Geometry: see drawing. Coordinates: mm, zero at the bounding-box minimum. Coordinates: 2 decimals unless noted, no trailing zeros. Write each loop counter-clockwise with the first axis right and the second up, starting at its lowest first coordinate (ties: lowest second). Pieces come first, ordered by that corner, then holes. Notation, with made-up numbers: (-0.5, -33) - (40.5, -33) arc R20 cw to (40.5, -13) - close; hole circle Ø6 at (-35, -21.75). An arc over 180 degrees is marked (long way). Use a Markdown table: item, result. Add a question column.
Q1. Section query B-B (z = 1). Return the cut outline in (x, y) (1 decimal).
Q2. Section query A-A (z = 4). Return the cut outline in (x, y) (1 decimal), then the cut area to 3 significant figures.
Q3. Section query C-C (y = 2.25). Return the cut outline in (x, z).
Q4. Section query D-D (x = 1.5). Return the cut outline in (y, z), then the cut area to 3 significant figures.
Q5. Material intervals for probe 1 along X at (y, z) = (14.25, 7.5); probe 2 along X at (y, z) = (14, 1.5); probe 3 along Y at (x, z) = (17, 1) (1 decimal), sorted ascending. Write a range as from..to.
Q6. Mould query, pull axis X, two halves, no side actions, for the marked faces 1, 2 and 3. Classes: released by +X, released by -X, zero draft, split by the parting line, or undercut.
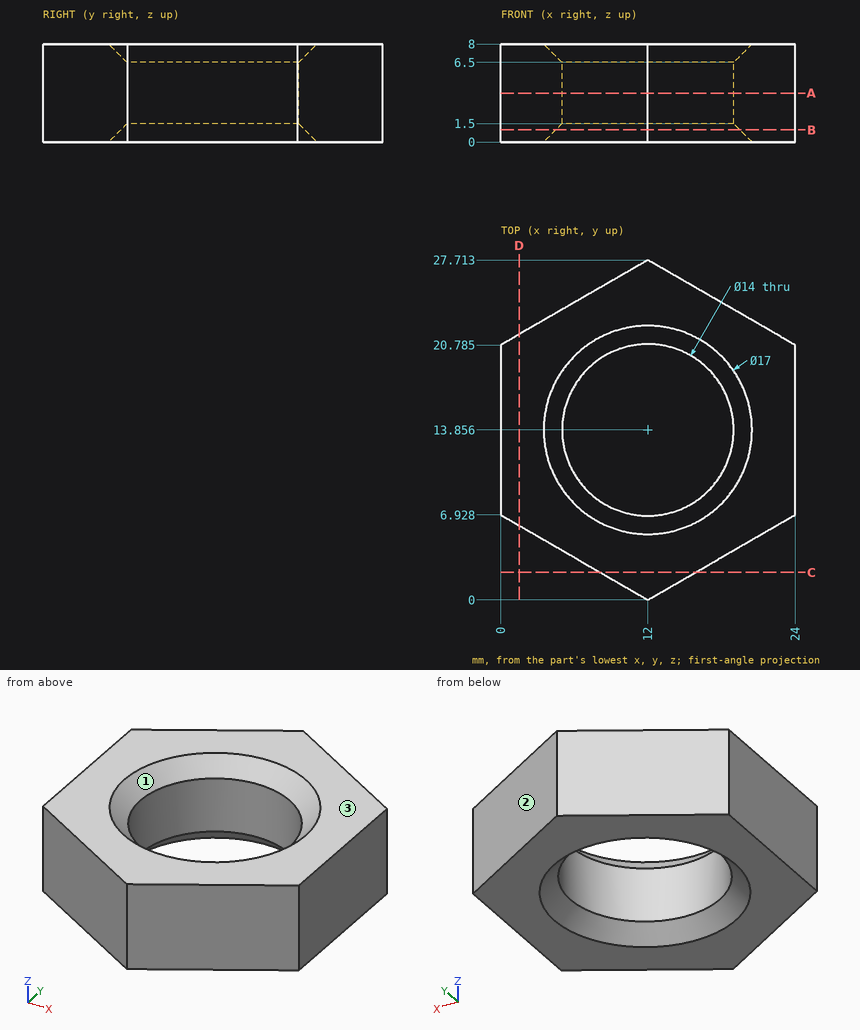
Values follow:
| question | item | result |
|---|---|---|
| 1 | outline | (0, 6.9) - (12, 0) - (24, 6.9) - (24, 20.8) - (12, 27.7) - (0, 20.8) - close; hole circle Ø15 at (12, 13.9) |
| 2 | outline | (0, 6.9) - (12, 0) - (24, 6.9) - (24, 20.8) - (12, 27.7) - (0, 20.8) - close; hole circle Ø14 at (12, 13.9) |
| 2 | area | 345 mm2 |
| 3 | outline | (8.1, 0) - (15.9, 0) - (15.9, 8) - (8.1, 8) - close |
| 4 | outline | (6.06, 0) - (21.65, 0) - (21.65, 8) - (6.06, 8) - close |
| 4 | area | 125 mm2 |
| 5 | probe 1 | 0..4.01, 19.99..24 |
| 5 | probe 2 | 0..5, 19..24 |
| 5 | probe 3 | 2.9..8.3, 19.4..24.8 |
| 6 | face 1 | undercut |
| 6 | face 2 | released by +X |
| 6 | face 3 | zero draft |
